Verification items for the finished model (mm, model axes). Face numbers are marked on the shaded views. A direction names the side the tool comes from. Give positions to 0.01 mm unless a question says otherwise; leave off trailing zeros. Write each loop counter-clockwise with the first axis right and the second up, starting at its lowest first coordinate (ties: lowest second). Pieces come first, ordered by that corner, then holes. Notation, with made-up numbers: M 53.5,85 L 79.5,85 A9 cw 79.5,100 Z; hole C 42,71.25 d7. An arc over 180 degrees is marked long. Answer as a JSON object with one key per item and string values.
Autodesk Inventor part; units mm, degrees
ref_plane "YZ Plane" through (0, 0, 0) normal (1, 0, 0) x (0, 1, 0)
ref_plane "XZ Plane" through (0, 0, 0) normal (0, 1, 0) x (-1, 0, 0)
ref_plane "XY Plane" through (0, 0, 0) normal (0, 0, 1) x (1, 0, 0)
sketch "Sketch1" plane through (0, 0, 0) normal (0, 0, 1) x (1, 0, 0)
  line L0 (0, 0) -> (160, 0)
  line L1 (160, 0) -> (118.589, -154.5481) construction
  line L2 (0, 0) -> (41.411, -154.5481) construction
  line L3 (41.411, -154.5481) -> (118.589, -154.5481)
  circle A0 centre (235.8871, -103.156) radius 80 construction
  line L4 (160, 0) -> (256.5926, -25.8819)
  line L5 (118.589, -154.5481) -> (215.1815, -180.43)
  arc A1 (215.1815, -180.43) -> (256.5926, -25.8819) centre (235.8871, -103.156) ccw
  circle A2 centre (-75.8871, -103.156) radius 80 construction
  line L6 (0, 0) -> (-96.5926, -25.8819)
  line L7 (41.411, -154.5481) -> (-55.1815, -180.43)
  arc A3 (-96.5926, -25.8819) -> (-55.1815, -180.43) centre (-75.8871, -103.156) ccw
  dimension "d0" = 160
  dimension "d1" = 160
  dimension "d2" = 160
  dimension "d3" = 75
  dimension "d4" = 75
  dimension "d5" = 160
  dimension "d6" = 100
  dimension "d7" = 160
  dimension "d9" = 100
extrude "Extrusion1" add sketch "Sketch1" along normal blind 33.9
sketch "Sketch2" plane through (0, 0, 33.9) normal (0, 0, 1) x (1, 0, 0)
  line L0 (-26.5, -133) -> (186.5, -133)
  line L1 (186.5, -133) -> (186.5, -20)
  line L2 (186.5, -20) -> (-26.5, -20)
  line L3 (-26.5, -20) -> (-26.5, -133)
  line L4 (160, 0) -> (0, 0)
  point P0 (80, -20)
  point P1 (80, 0)
  dimension "d12" = 213
  dimension "d13" = 113
  dimension "d14" = 20
extrude "Extrusion2" cut sketch "Sketch2" against normal through all
sketch "Sketch3" plane through (0, 0, 33.9) normal (0, 0, 1) x (1, 0, 0)
  line L0 (-26.5, -133) -> (-26.5, -20) construction
  line L1 (-26.5, -20) -> (186.5, -20) construction
  line L2 (186.5, -20) -> (186.5, -133) construction
  line L3 (186.5, -133) -> (-26.5, -133) construction
  line L4 (-48.0481, 1.5481) -> (-48.0481, -154.5481) construction
  line L5 (-48.0481, -154.5481) -> (208.0481, -154.5481) construction
  line L6 (208.0481, -154.5481) -> (208.0481, 1.5481) construction
  line L7 (208.0481, 1.5481) -> (-48.0481, 1.5481) construction
  line L8 (41.411, -154.5481) -> (118.589, -154.5481) construction
  line L9 (-48.0481, 1.5481) -> (-48.0481, -178.5186) construction
  line L10 (-55.1815, -180.43) -> (41.411, -154.5481) construction
  line L11 (208.0481, 1.5481) -> (208.0481, -178.5186) construction
  line L12 (118.589, -154.5481) -> (215.1815, -180.43) construction
  line L13 (-48.0481, -178.5186) -> (208.0481, -178.5186) construction
  line L14 (-48.0481, 1.5481) -> (208.0481, 1.5481) construction
  line L15 (160, 0) -> (256.5926, -25.8819) construction
  line L16 (208.2963, -12.941) -> (208.0481, -178.5186)
  line L17 (208.2963, -12.941) -> (256.5926, -25.8819)
  line L18 (208.0481, -178.5186) -> (215.1815, -180.43)
  arc A0 (215.1815, -180.43) -> (256.5926, -25.8819) centre (235.8871, -103.156) ccw
  line L19 (208.0481, 1.5481) -> (-166.9519, 1.5481)
  line L20 (-166.9519, 1.5481) -> (-166.9519, -188.4519)
  line L21 (-166.9519, -188.4519) -> (208.0481, -188.4519)
  line L22 (208.0481, -188.4519) -> (208.0481, 1.5481)
  point P0 (0, 0)
  point P1 (80, -154.5481)
  dimension "d17" = 190
  dimension "d18" = 375
extrude "Extrusion3" cut sketch "Sketch3" against normal through all contours L22 L21 L20 L19
sketch "Sketch4" plane through (0, 0, 33.9) normal (0, 0, 1) x (1, 0, 0)
  arc A0 (215.1815, -180.43) -> (256.5926, -25.8819) centre (235.8871, -103.156) ccw
  circle A1 centre (235.8871, -103.156) radius 6.5
  point P0 (0, 0)
  dimension "d21" = 13
extrude "Extrusion4" cut sketch "Sketch4" against normal through all
sketch "Sketch5" plane through (208.0481, -178.5186, 33.9) normal (-1, 0, 0) x (0, 0, 1)
  line L0 (-33.9, 165.6442) -> (0, 165.6442)
  line L1 (-33.9, 0) -> (-33.9, 165.6442)
  line L2 (0, 0) -> (-33.9, 0)
  line L3 (0, 165.6442) -> (0, 0)
  line L4 (-25.4, 157.1442) -> (-8.5, 157.1442)
  line L5 (-8.5, 157.1442) -> (-8.5, 8.5)
  line L6 (-8.5, 8.5) -> (-25.4, 8.5)
  line L7 (-25.4, 8.5) -> (-25.4, 157.1442)
  point P0 (-33.9, 178.5186)
  dimension "d24" = 8.5
extrude "Extrusion5" add sketch "Sketch5" along normal blind 13 contours L4 L5 L6 L7
sketch "Sketch6" plane through (208.0481, -170.0186, 8.5) normal (0, 0, -1) x (-1, 0, 0)
  circle A0 centre (8, 74.3221) radius 2.5
  line L0 (0, -8.5) -> (0, 157.1442)
  point P0 (208.0481, 170.0186)
  point P1 (0, 74.3221)
  dimension "d27" = 5
  dimension "d28" = 8
extrude "Extrusion6" cut sketch "Sketch6" against normal through all
sketch "Sketch7" plane through (0, 0, 0) normal (0, 0, -1) x (-1, 0, 0)
  circle A0 centre (-235.8871, -103.156) radius 6.5
  line L0 (-208.0481, -178.5186) -> (-208.0481, -12.8745)
  line L1 (-208.0481, -12.8745) -> (-256.5926, -25.8819)
  arc A1 (-256.5926, -25.8819) -> (-215.1815, -180.43) centre (-235.8871, -103.156) ccw
  line L2 (-215.1815, -180.43) -> (-208.0481, -178.5186)
  line L3 (-254.522, -33.6093) -> (-216.0481, -23.3003)
  line L4 (-216.0481, -23.3003) -> (-216.0481, -172.38)
  line L5 (-216.0481, -172.38) -> (-217.2521, -172.7026)
  arc A2 (-254.522, -33.6093) -> (-217.2521, -172.7026) centre (-235.8871, -103.156) ccw
  circle A3 centre (-235.8871, -103.156) radius 14.5
  point P0 (0, 0)
  dimension "d31" = 8
  dimension "d32" = 8
extrude "Extrusion7" cut sketch "Sketch7" against normal through all contours L3 L4 L5 A2
sketch "Sketch8" plane through (0, 0, 0) normal (0, 0, -1) x (-1, 0, 0)
  circle A0 centre (-235.8871, -103.156) radius 6.5 construction
  circle A1 centre (-235.8871, -103.156) radius 14.5 construction
  line L0 (-235.8871, -103.156) -> (-159.7277, -103.156) construction
  line L1 (-222.2764, -98.156) -> (-123.6167, -98.156) construction
  line L2 (-222.2764, -108.156) -> (-123.6167, -108.156) construction
  line L3 (-233.4119, -88.8688) -> (-184.082, -3.427) construction
  line L4 (-224.7516, -93.8688) -> (-175.4217, -8.427) construction
  line L5 (-247.0225, -93.8688) -> (-296.3524, -8.427) construction
  line L6 (-238.3623, -88.8688) -> (-287.6921, -3.427) construction
  line L7 (-249.4977, -108.156) -> (-348.1575, -108.156) construction
  line L8 (-249.4977, -98.156) -> (-348.1575, -98.156) construction
  line L9 (-238.3623, -117.4431) -> (-287.6921, -202.885) construction
  line L10 (-247.0225, -112.4431) -> (-296.3524, -197.885) construction
  line L11 (-224.7516, -112.4431) -> (-175.4217, -197.885) construction
  line L12 (-233.4119, -117.4431) -> (-184.082, -202.885) construction
  line L13 (-216.0481, -23.3003) -> (-216.0481, -172.38) construction
  arc A2 (-254.522, -33.6093) -> (-217.2521, -172.7026) centre (-235.8871, -103.156) ccw construction
  line L14 (-254.522, -33.6093) -> (-216.0481, -23.3003) construction
  line L15 (-216.0481, -172.38) -> (-217.2521, -172.7026) construction
  line L16 (-222.2764, -98.156) -> (-216.0481, -98.156)
  line L17 (-222.2764, -108.156) -> (-216.0481, -108.156)
  line L18 (-224.7516, -112.4431) -> (-216.0481, -127.518)
  line L19 (-233.4119, -117.4431) -> (-216.0481, -147.518)
  line L20 (-238.3623, -117.4431) -> (-267.47, -167.8593)
  line L21 (-276.1303, -162.8593) -> (-247.0225, -112.4431)
  line L22 (-249.4977, -108.156) -> (-307.7132, -108.156)
  line L23 (-249.4977, -98.156) -> (-307.7132, -98.156)
  line L24 (-247.0225, -93.8688) -> (-276.1303, -43.4527)
  line L25 (-238.3623, -88.8688) -> (-267.47, -38.4527)
  line L26 (-233.4119, -88.8688) -> (-216.0481, -58.7939)
  line L27 (-224.7516, -93.8688) -> (-216.0481, -78.7939)
  line L28 (-216.0481, -58.7939) -> (-216.0481, -78.7939)
  line L29 (-216.0481, -98.156) -> (-216.0481, -108.156)
  line L30 (-216.0481, -127.518) -> (-216.0481, -147.518)
  arc A3 (-267.47, -38.4527) -> (-276.1303, -43.4527) centre (-235.8871, -103.156) ccw
  arc A4 (-307.7132, -98.156) -> (-307.7132, -108.156) centre (-235.8871, -103.156) ccw
  arc A5 (-276.1303, -162.8593) -> (-267.47, -167.8593) centre (-235.8871, -103.156) ccw
  arc A6 (-222.2764, -108.156) -> (-222.2764, -98.156) centre (-235.8871, -103.156) ccw
  arc A7 (-233.4119, -117.4431) -> (-224.7516, -112.4431) centre (-235.8871, -103.156) ccw
  arc A8 (-247.0225, -112.4431) -> (-238.3623, -117.4431) centre (-235.8871, -103.156) ccw
  arc A9 (-249.4977, -98.156) -> (-249.4977, -108.156) centre (-235.8871, -103.156) ccw
  arc A10 (-238.3623, -88.8688) -> (-247.0225, -93.8688) centre (-235.8871, -103.156) ccw
  arc A11 (-224.7516, -93.8688) -> (-233.4119, -88.8688) centre (-235.8871, -103.156) ccw
  point P0 (0, 0)
  dimension "d36" = 5
  dimension "d37" = 5
  dimension "d40" = 360
extrude "Extrusion8" add sketch "Sketch8" against normal blind 33.9
properties part number "Riser Base" material "ABS Plastic"
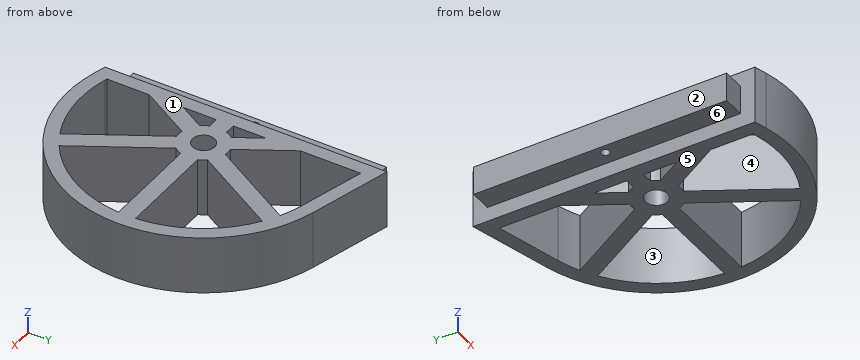
1) Thickness scan on L1, parallel to Y at x = 282.5, z = 17; L2, parallel to X at y = -161, z = 11; L3, parallel to Y at x = 243.5, z = 1. Record the ranges inside material, lowest first.
Completed:
{"L1": "y = -168.17 to -158.03, -108.16 to -98.16, -48.28 to -38.14", "L2": "x = 195.05 to 216.05, 263.51 to 275.06, 278.76 to 291.15", "L3": "y = -182.79 to -174.75, -126.34 to -79.97, -30.66 to -22.37"}
2) Section check B-B on x = 289.5. Record the boundary of the cut face in (y, z), and give its area (3 significant figures).
Completed:
{"outline": "M -162.53,0 L -151.21,0 L -151.21,33.9 L -162.53,33.9 Z; M -108.16,0 L -98.16,0 L -98.16,33.9 L -108.16,33.9 Z; M -55.1,0 L -43.78,0 L -43.78,33.9 L -55.1,33.9 Z", "area": "1,110 mm2"}
3) Section check A-A on y = -115. Record the boundary of the cut face in (x, z), and give its area (3 significant figures).
Completed:
{"outline": "M 195.05,8.5 L 208.05,8.5 L 208.05,0 L 216.05,0 L 216.05,33.9 L 208.05,33.9 L 208.05,25.4 L 195.05,25.4 Z; M 223.28,0 L 248.5,0 L 248.5,33.9 L 223.28,33.9 Z; M 306.91,0 L 315.01,0 L 315.01,33.9 L 306.91,33.9 Z", "area": "1,620 mm2"}
4) Release check for a two-part mould opening along X. For the marked faces 1, 2 and 3 record: pulls with the +X half, pulls with the -X half, needs draft (parallel to the pull), parting line crosses it, or undercut.
Completed:
{"face 1": "needs draft", "face 2": "pulls with the -X half", "face 3": "undercut"}
5) Go/stop test with flat-tipped pins: pin 1 (12.5 mm diameter, centred on y = -157, z = 24.5, fed in from +X); pin 2 (10.5 mm diameter, centred on x = 203, z = 18.5, fed in from +Y); pin 3 (6.5 mm diameter, centred on x = 201, y = -63.5, fed in from +Z); pin 4 (12 mm diameter, centred on x = 233.5, y = -36, fed in from -Z). Record where each tip stops, or that it passes through.
Completed:
{"pin 1": "stops at x = 300.19", "pin 2": "stops at y = -12.87", "pin 3": "stops at z = 25.4", "pin 4": "passes through"}
6) Section check C-C on z = 30. Count the separate pieces of the cut face and the enclosed holes in it, and give its area (3 significant figures).
Completed:
{"separate pieces": "1", "enclosed holes": "7", "area": "6,390 mm2"}
7) Access from +Z, -Z, +X, -X, +Y, -Y to the whole of each face (thin tool, end or side, straight path). Record for the marked faces 4, 5 and 6.
Completed:
{"face 4": "+Z, -Z", "face 5": "-Z, +X, -X, +Y, -Y", "face 6": "-Z, -X, +Y, -Y"}
8) Section check D-D on y = -86.5. Record the boundary of the cut face in (x, z).
Completed:
{"outline": "M 195.05,8.5 L 208.05,8.5 L 208.05,0 L 216.05,0 L 216.05,33.9 L 208.05,33.9 L 208.05,25.4 L 195.05,25.4 Z; M 220.5,0 L 232.04,0 L 232.04,33.9 L 220.5,33.9 Z; M 239.73,0 L 251.28,0 L 251.28,33.9 L 239.73,33.9 Z; M 305.93,0 L 314.13,0 L 314.13,33.9 L 305.93,33.9 Z"}
